Here's how the part is built. I have some questions about the finished solid (model axes, mm). A direction names the side the tool comes from. Give positions to 0.01 mm unless a question says otherwise; leave off trailing zeros. Loops run counter-clockwise (first coordinate to the right, second up) from the corner with the lowest first, then second, coordinate; pieces in that order, holes last.
Q1. I need wall thicknesses on line 1 (Z direction, x = 0.75, y = -13.25); line 2 (X direction, y = -8.75, z = 1.65); line 3 (Z direction, x = -4.5, y = -11.5). Which ranges of each line are inside material? Lowest first, please.
Q2. For faces 1 (the face through (6, -11, 0)), 2 (the face through (0, -12, 2)), which set-ups out of +Z, -Z, +X, -X, +Y, -Y let a thin tool reach every point of the face, with its end or its side?
Q3. If we section it at C-C (z = -0.9): Please give me the cut outline in (x, y).
Q4. Will this pin go through, and if not, where does the flat tip stop? P1, Ø1, axis at x = 4.5, z = 2, coming from the +Y side.
Q5. If we section it at B-B (y = -7): Please give me the cut outline in (x, z), plus the area to 3 significant figures.
Q6. We'd pull the mould along X, two halves only. Please class faces 3 (the face through (5.5, -12, 0)), 4 (the face through (-6, -11, 0)), 5 (the face through (-5.5, -12, 0)), 6 (the face through (0, 0, 0)): +X half, -X half, draft (parallel to the pull), parting line (faces both ways), or undercut.
Q7. If we section it at A-A (x = 3.5): Please give me the cut outline in (y, z).
from build123d import *

# Parameters (mm, degrees)
F0_W     = 12
F0_H     = 5
F1_DEPTH = 23
F2_T     = -0.5
F3_W     = 3
F3_H     = 3
F4_DEPTH = 4.2
F5_W     = 3
F5_H     = 3
F6_DEPTH = 6.2


with BuildPart() as f1:
    # F0 (on Front) → F1 (new body)
    with BuildSketch(Plane.XZ):
        Rectangle(F0_W, F0_H)
    extrude(amount=F1_DEPTH)

    # F2
    f2_openings = [f1.faces().sort_by_distance(p)[0] for p in [
        (0, -23, 0),
    ]]
    offset(amount=F2_T, openings=f2_openings)

    # F3 (on Top) → F4 (cut)
    with BuildSketch(Plane.XY):
        with Locations((-3.345713, -11.96193)):
            Rectangle(F3_W, F3_H)
    extrude(amount=F4_DEPTH, mode=Mode.SUBTRACT)

    # F5 (on Top) → F6 (cut)
    with BuildSketch(Plane.XY):
        with Locations((3.351791, -12.00388)):
            Rectangle(F5_W, F5_H)
    extrude(amount=F6_DEPTH, mode=Mode.SUBTRACT)


solid = f1.part
Check sheet entries:
1. line 1: z = -2.5 to -2, 2 to 2.5
1. line 2: x = -6 to -5.5, 5.5 to 6
1. line 3: z = -2.5 to -2
2. face 1: +Z, -Z, +X, +Y, -Y
2. face 2: -Y
3. outline: (-6, -23) - (-5.5, -23) - (-5.5, -0.5) - (5.5, -0.5) - (5.5, -23) - (6, -23) - (6, 0) - (-6, 0) - close
4. P1: stops at y = 0
5. outline: (-6, -2.5) - (6, -2.5) - (6, 2.5) - (-6, 2.5) - close; hole (-5.5, -2) - (5.5, -2) - (5.5, 2) - (-5.5, 2) - close
5. area: 16.0 mm2
6. face 3: undercut
6. face 4: -X half
6. face 5: undercut
6. face 6: draft
7. outline: (-23, -2.5) - (0, -2.5) - (0, 2.5) - (-10.5, 2.5) - (-10.5, 2) - (-0.5, 2) - (-0.5, -2) - (-23, -2) - close; (-23, 2) - (-13.5, 2) - (-13.5, 2.5) - (-23, 2.5) - close
